Autodesk Inventor part; units mm, degrees
ref_plane "YZ Plane" through (0, 0, 0) normal (1, 0, 0) x (0, 1, 0)
ref_plane "XZ Plane" through (0, 0, 0) normal (0, 1, 0) x (-1, 0, 0)
ref_plane "XY Plane" through (0, 0, 0) normal (0, 0, 1) x (1, 0, 0)
sketch "Sketch3" plane through (0, 0, 0) normal (1, 0, 0) x (0, 1, 0)
  line L0 (23.8462, 26.7077) -> (8.4462, 26.7077) construction
  line L1 (8.4462, 26.7077) -> (8.4462, 14.3077)
  line L2 (8.4462, 14.3077) -> (23.8462, 14.3077) construction
  line L3 (23.8462, 14.3077) -> (23.8462, 26.7077)
  line L4 (16.1462, 26.7077) -> (16.1462, 30.7077) construction
  line L5 (16.1462, 14.3077) -> (16.1462, 10.3077) construction
  arc A0 (8.4462, 14.3077) -> (23.8462, 14.3077) centre (16.1462, 19.7189) ccw
  arc A1 (23.8462, 26.7077) -> (8.4462, 26.7077) centre (16.1462, 21.2964) ccw
  point P0 (0, 0)
  dimension "d9" = 12.4
  dimension "d10" = 15.4
  dimension "d11" = 4
  dimension "d12" = 4
  dimension "d13" = 20.4
extrude "Extrusion1" add sketch "Sketch3" along normal blind 25.1
sketch "Sketch4" plane through (0, 0, 0) normal (-1, 0, 0) x (0, 0, 1)
  line L0 (26.7077, 8.4462) -> (14.3077, 8.4462)
  line L1 (14.3077, 23.8462) -> (26.7077, 23.8462)
  arc A0 (14.3077, 23.8462) -> (14.3077, 8.4462) centre (19.7189, 16.1462) ccw
  arc A1 (26.7077, 8.4462) -> (26.7077, 23.8462) centre (21.2964, 16.1462) ccw
  circle A2 centre (20.5077, 16.1462) radius 3.075
  point P0 (0, 0)
  dimension "d16" = 6.15
extrude "Extrusion2" add sketch "Sketch4" along normal blind 1.6 contours A2
sketch "Sketch5" plane through (-1.6, 16.1462, 20.5077) normal (-1, 0, 0) x (0, 0, 1)
  circle A0 centre (0, 0) radius 1
  point P0 (-20.5077, -16.1462)
  dimension "d19" = 2
extrude "Extrusion3" add sketch "Sketch5" along normal blind 9.95
fillet "Fillet3" radius 1 5 edges at (-1.6, 16.1462, 17.4327) (0, 23.8462, 20.5077) (0, 16.1462, 30.7077) (0, 8.4462, 20.5077) (0, 16.1462, 10.3077)
properties part number "Motor" material "Iron, Cast"
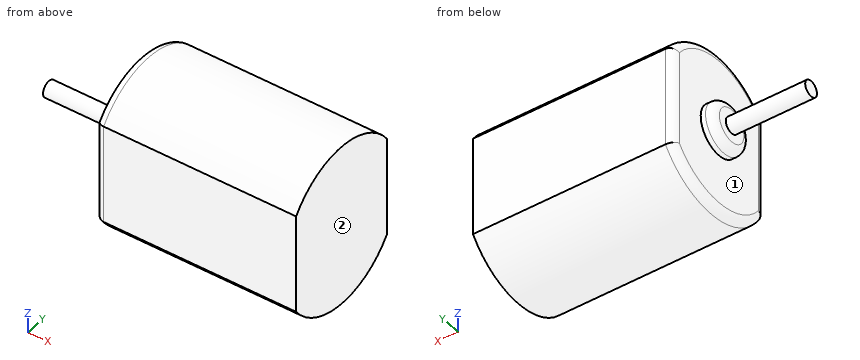
The model under review builds one solid part; all positions refer to its coordinate system, in mm. Face numbers are marked on the shaded views. A direction names the side the tool comes from. Give positions to 0.01 mm unless a question says otherwise; leave off trailing zeros. Write each loop counter-clockwise with the first axis right and the second up, starting at its lowest first coordinate (ties: lowest second). Pieces come first, ordered by that corner, then holes.
(1) For P1, Ø2, axis at y = 15, z = 26, coming from the -X side; P2, Ø1, axis at x = 15, y = 13, coming from the +Z side, all flat-tipped, find the tip position at first contact; note any pin that passes through.
(2) Consider section A-A, the plane z = 24. Give the boundary of the cut face in (x, y).
(3) To check wall thickness, follow L1, parallel to Z at x = 3.5, y = 16.25; L2, parallel to X at y = 20.5, z = 18.75; L3, parallel to X at y = 15.5, z = 18.5. State the ranges of each line that lie inside material, in increasing order.
(4) Tool access review of the marked faces 1 and 2: name each direction out of +Z, -Z, +X, -X, +Y, -Y from which nothing blocks a thin tool from reaching the whole face with its end or side.
(5) Consider section C-C, the plane x = -1. Give the boundary of the cut face in (y, z), and give its area (3 significant figures).
(6) Consider section B-B, the plane x = 23.5. Give the boundary of the cut face in (y, z), and give its area (3 significant figures).
Returned:
1. P1: stops at x = 0
1. P2: stops at z = 30.33
2. outline: (0, 9.45) arc R1 ccw to (1, 8.45) - (25.1, 8.45) - (25.1, 23.85) - (1, 23.85) arc R1 ccw to (0, 22.85) - close
3. L1: z = 10.31 to 30.71
3. L2: x = 0 to 25.1
3. L3: x = -1.6 to 25.1
4. face 1: -X
4. face 2: +Z, -Z, +X, +Y, -Y
5. outline: circle Ø5.98 at (16.15, 20.51)
5. area: 28.1 mm2
6. outline: (8.45, 14.31) arc R9.41 ccw to (23.85, 14.31) - (23.85, 26.71) arc R9.41 ccw to (8.45, 26.71) - close
6. area: 277 mm2
